```python
from build123d import *

# Parameters (mm, degrees)
F0_W     = 38
F0_H     = 1.8
F0_R     = 1.6
F1_DEPTH = 50
F2_W     = 39.500002
F2_H     = 7.7
F2_H_2   = 13.4
F2_W_2   = 59.247335
F2_H_3   = 31.547058
F3_DEPTH = 25
F4_W     = 3
F4_H     = 8
F5_DEPTH = 1.8


with BuildPart() as f1:
    # F0 (on Top) → F1 (new body)
    with BuildSketch(Plane.XY):
        with Locations((-19, 0)):
            Rectangle(F0_W, F0_H)
        with BuildLine():
            add(Edge.make_bspline(
                [(0, 3.8), (0, 2.602653), (0.90178, 1.877582), (0, 0.9)],
                knots=[0, 0, 0, 0, 2.9, 2.9, 2.9, 2.9], degree=3))
            Line((0, 0.9), (0, -0.9))
            add(Edge.make_bspline(
                [(0, -0.9), (3.389107, -0.9), (5, -1.015936), (5, 3.8)],
                knots=[0, 0, 0, 0, 6.862215, 6.862215, 6.862215, 6.862215], degree=3))
            ThreePointArc((5, 3.8), (2.5, 6.3), (0, 3.8))
        make_face()
        with Locations((2.5, 3.8)):
            Circle(F0_R, mode=Mode.SUBTRACT)
    extrude(amount=F1_DEPTH)

    # F2 (on Right) → F3 (cut)
    with BuildSketch(Plane.YZ):
        with Locations((1.306903, 3.85)):
            Rectangle(F2_W, F2_H)
        with Locations((0.349251, 25)):
            Rectangle(F2_W, F2_H_2)
        with Locations((-2.001637, 58.073529)):
            Rectangle(F2_W_2, F2_H_3)
    extrude(amount=F3_DEPTH, mode=Mode.SUBTRACT)

    # F4 (on face) → F5 (cut, through all)
    with BuildSketch(Plane.XZ.offset(0.9)):
        with Locations((-32.5, 25)):
            Rectangle(F4_W, F4_H)
        with Locations((-26.5, 25)):
            Rectangle(F4_W, F4_H)
        with Locations((-14.5, 25)):
            Rectangle(F4_W, F4_H)
        with Locations((-8.5, 25)):
            Rectangle(F4_W, F4_H)
    extrude(amount=-F5_DEPTH, mode=Mode.SUBTRACT)


solid = f1.part
```
Geometry check sheet. Reference: the model listing, model coordinates, mm. A direction names the side the tool comes from. Coordinates: 2 decimals unless noted, no trailing zeros. Write each loop counter-clockwise with the first axis right and the second up, starting at its lowest first coordinate (ties: lowest second). Pieces come first, ordered by that corner, then holes. Notation, with made-up numbers: M 55.5,48.5 L 93.5,48.5 A19 ccw 93.5,65.5 Z; hole C 84,71 d8. An arc over 180 degrees is marked long. One line per item, written item: value. Start each with the question number.
(1) Tool access check on faces 1 (the face through (0, 0, 46)), 2 (the face through (2, 2, 7.7)), 3 (the face through (0, 0, 25)), 4 (the face through (-27, 0, 21)). Record the directions out of +Z, -Z, +X, -X, +Y, -Y that give a thin tool (end or side, any length) a straight path to the whole face; none if there is none.
(2) Sectioned sample at B-B, the plane x = -8.5. Enter the section's corners in (y, z), and give its area (3 significant figures).
(3) Sectioned sample at D-D, the plane x = 2.5. State how many separate pieces and enclosed holes the cut face has, and give its area (3 significant figures).
(4) Sectioned sample at A-A, the plane z = 23.5. Enter the section's corners in (x, y), and give its area (3 significant figures).
(5) Scan lines: line 1 along Z through (x, y) = (2, 0); line 2 along X through (y, z) = (3.8, 14.25); line 3 along Y through (x, z) = (2.5, 12.25). Record each from-to range of solid material in increasing order. Write a range as [from, to].
(6) Sectioned sample at C-C, the plane y = 4.75. Enter the section's corners in (x, z).
(7) Release check for a two-part mould opening along Z. For faces 5 (the face through (-27, 0, 29)), 6 (the face through (0, 0, 4)), 7 (the face through (-19, 0, 50)) record: released by +Z, released by -Z, zero draft, split by the parting line, or undercut.
(8) Depth check by flat-ended pin: pin 1 (0.9 mm diameter, centred on y = 0, z = 24.5, fed in from +X); pin 2 (2.5 mm diameter, centred on x = 3, y = 1.5, fed in from +Z); pin 3 (4 mm diameter, centred on y = 3, z = 28, fed in from -X); pin 4 (2 mm diameter, centred on x = -19, z = 16, fed in from +Y). Enter the tip coordinate at first touch or a pass-through.
Filled sheet:
1. face 1: +Z, +X, +Y, -Y
1. face 2: -Z, +X, +Y, -Y
1. face 3: +X, +Y, -Y
1. face 4: +Y, -Y
2. outline: M -0.9,0 L 0.9,0 L 0.9,21 L -0.9,21 Z; M -0.9,29 L 0.9,29 L 0.9,50 L -0.9,50 Z
2. area: 75.6 mm²
3. separate pieces: 4
3. enclosed holes: 0
3. area: 82.8 mm²
4. outline: M -38,-0.9 L -34,-0.9 L -34,0.9 L -38,0.9 Z; M -31,-0.9 L -28,-0.9 L -28,0.9 L -31,0.9 Z; M -25,-0.9 L -16,-0.9 L -16,0.9 L -25,0.9 Z; M -13,-0.9 L -10,-0.9 L -10,0.9 L -13,0.9 Z; M -7,-0.9 L 0,-0.9 L 0,0.9 L -7,0.9 Z
4. area: 46.8 mm²
5. line 1: [7.7, 18.3], [31.7, 42.3]
5. line 2: [0, 0.9], [4.1, 5]
5. line 3: [-0.81, 2.2], [5.4, 6.3]
6. outline: M 0.19,7.7 L 1.21,7.7 L 1.21,18.3 L 0.19,18.3 Z; M 0.19,31.7 L 1.21,31.7 L 1.21,42.3 L 0.19,42.3 Z; M 3.79,7.7 L 4.81,7.7 L 4.81,18.3 L 3.79,18.3 Z; M 3.79,31.7 L 4.81,31.7 L 4.81,42.3 L 3.79,42.3 Z
7. face 5: undercut
7. face 6: zero draft
7. face 7: released by +Z
8. pin 1: x = 0
8. pin 2: z = 42.3
8. pin 3: through
8. pin 4: y = 0.9
